Geometry: final body of the model. Coordinates: model frame, mm. A direction names the side the tool comes from. Give positions to 0.01 mm unless a question says otherwise; leave off trailing zeros. Order: outer loops, then holes, each group sorted by start corner. A loop starts at its lowest first (then second) coordinate and runs counter-clockwise, first axis right, second up. Notation, with made-up numbers: M 67.5,-24.75 L 103.5,-24.75 A21 ccw 103.5,1.25 Z; hole C 46.5,-6 d11. An arc over 180 degrees is marked long. One line per item, written item: value. Start each with the question number.
Autodesk Inventor part; units mm, degrees
ref_plane "YZ Plane" through (0, 0, 0) normal (1, 0, 0) x (0, 1, 0)
ref_plane "XZ Plane" through (0, 0, 0) normal (0, 1, 0) x (-1, 0, 0)
ref_plane "XY Plane" through (0, 0, 0) normal (0, 0, 1) x (1, 0, 0)
sketch "スケッチ1" plane through (0, 0, 0) normal (0, 0, 1) x (1, 0, 0)
  line L0 (0, 18.2674) -> (0, -9.7942)
  line L1 (0, -4.65) -> (-2.5, -4.65)
  line L2 (-2.5, -4.65) -> (-2.5, -6.65)
  line L3 (-2.5, -6.65) -> (-3.5, -6.65)
  line L4 (-10.8284, 8.5) -> (-4.8284, 8.5)
  line L5 (-4.8284, 8.5) -> (-4.8284, 3.5)
  line L6 (-4.8284, 3.5) -> (-7.8284, 3.5)
  line L7 (-7.8284, 3.5) -> (-3.5, -6.65)
  line L8 (-10.8284, 8.5) -> (-10.8284, 10)
  line L9 (-10.8284, 10) -> (-2.5, 11.5)
  line L10 (-2.5, 11.5) -> (-2.5, 5.5)
  line L11 (-2.5, 5.5) -> (0, 5.5)
  line L12 (0, -4.65) -> (2.5, -4.65)
  line L13 (2.5, -4.65) -> (2.5, -6.65)
  line L14 (2.5, -6.65) -> (3.5, -6.65)
  line L15 (10.8284, 8.5) -> (4.8284, 8.5)
  line L16 (4.8284, 8.5) -> (4.8284, 3.5)
  line L17 (4.8284, 3.5) -> (7.8284, 3.5)
  line L18 (7.8284, 3.5) -> (3.5, -6.65)
  line L19 (10.8284, 8.5) -> (10.8284, 10)
  line L20 (10.8284, 10) -> (2.5, 11.5)
  line L21 (2.5, 11.5) -> (2.5, 5.5)
  line L22 (2.5, 5.5) -> (0, 5.5)
  line L23 (-2.8284, 0) -> (0, 2.8284)
  line L24 (0, 2.8284) -> (2.8284, 0)
  line L25 (2.8284, 0) -> (0, -2.8284)
  line L26 (0, -2.8284) -> (-2.8284, 0)
  point P0 (0, 0)
  point P1 (0, 3.5)
  point P2 (0, -2.65)
  point P3 (2.8284, 0)
  dimension "d23" = 2
  dimension "d31" = 1
  dimension "d33" = 2
  dimension "d34" = 6
  dimension "d35" = 3
  dimension "d39" = 5
  dimension "d41" = 3
  dimension "d42" = 5
  dimension "d43" = 5
  dimension "d44" = 2
  dimension "d45" = 1.5
  dimension "d46" = 2
  dimension "d50" = 4
  dimension "d51" = 3.5
extrude "押し出し1" add sketch "スケッチ1" along normal blind 40 contours L22 L21 L20 L19 L15 L16 L17 L18 L14 L13 L12 L0 L25 L24 | L0 L23 L26 L1 L2 L3 L7 L6 L5 L4 L8 L9 L10 L11
fillet "フィレット2" radius 1 4 edges at (-3.5, -6.65, 20) (3.5, -6.65, 20) (10.8284, 10, 20) (-10.8284, 10, 20)
properties part number "TailRod_N_o" material "ABS プラスチック"
Q1. Contact query for flat-ended pins moving along their axis: pin 1 (2 mm diameter, centred on y = -5, z = 18.5, fed in from +X); pin 2 (3 mm diameter, centred on x = 8, z = 30, fed in from -Y); pin 3 (0.6 mm diameter, centred on y = -6, z = 23.5, fed in from -X). Output: stop coordinate, or through.
Q2. Section query A-A on y = 8. Return loops of the section in (x, z), and give its area (3 significant figures).
Q3. Section query B-B on z = 28. Return loops of the section in (x, y).
Q4. Ray query, line 1 along X through (y, z) = (5.75, 4.5); line 2 along Y through (x, z) = (-5.25, 28.5); line 3 along Y through (x, z) = (7.5, 26). Return the intervals inside material, ascending. Write a range as [from, to].
Q5. Set-up query: faces 4 (the face through (0, 5.5, 20)), 5 (the face through (-1.394, -1.434, 19.72)), 6 (the face through (4.828, 6, 20)), 7 (the face through (-8, 8.5, 20)), 8 (the face through (6.305, 10.815, 19.72)). Return all of +Z, -Z, +X, -X, +Y, -Y with unobstructed straight access to the full face (end or side cutting, diameter ignored); none if empty.
Q6. Section query C-C on x = -6.5. Return loops of the section in (y, z), and give its area (3 significant figures).
Q7. Section query D-D on y = 5. Return loops of the section in (x, z), and give its area (3 significant figures).
Q8. Mould query, pull axis X, two halves, no side actions, for faces 1 (the face through (0, 5, 40)), 2 (the face through (2.5, -6, 20)), 3 (the face through (-6.305, 10.815, 19.72)). Classes: +X half, -X half, draft (parallel to the pull), parting line (faces both ways), or undercut.
Results below:
1. pin 1: x = 4.63
1. pin 2: y = 0.38
1. pin 3: x = -3.91
2. outline: M -4.83,0 L -2.5,0 L -2.5,40 L -4.83,40 Z; M 2.5,0 L 4.83,0 L 4.83,40 L 2.5,40 Z
2. area: 186 mm2
3. outline: M -10.83,8.5 L -4.83,8.5 L -4.83,3.5 L -7.83,3.5 L -3.76,-6.04 A1 ccw -2.84,-6.65 L -2.5,-6.65 L -2.5,-4.65 L 2.5,-4.65 L 2.5,-6.65 L 2.84,-6.65 A1 ccw 3.76,-6.04 L 7.83,3.5 L 4.83,3.5 L 4.83,8.5 L 10.83,8.5 L 10.83,9.16 A1 ccw 10.01,10.15 L 2.5,11.5 L 2.5,5.5 L -2.5,5.5 L -2.5,11.5 L -10.01,10.15 A1 ccw -10.83,9.16 Z; hole M -2.83,0 L 0,-2.83 L 2.83,0 L 0,2.83 Z
4. line 1: [-4.83, -2.5], [2.5, 4.83]
4. line 2: [-2.55, 3.5], [8.5, 11]
4. line 3: [2.73, 3.5], [8.5, 10.6]
5. face 4: +Z, -Z, +Y
5. face 5: +Z, -Z
5. face 6: +Z, -Z, +X
5. face 7: +Z, -Z, -X
5. face 8: +Z, -Z, +X, +Y
6. outline: M 0.38,0 L 3.5,0 L 3.5,40 L 0.38,40 Z; M 8.5,0 L 10.78,0 L 10.78,40 L 8.5,40 Z
6. area: 216 mm2
7. outline: M -4.83,0 L 4.83,0 L 4.83,40 L -4.83,40 Z
7. area: 386 mm2
8. face 1: draft
8. face 2: undercut
8. face 3: -X half
